For this review, take the finished solid that the model builds, in its own axes (mm). Face numbers are marked on the shaded views. A direction names the side the tool comes from. Coordinates: 2 decimals unless noted, no trailing zeros. Write each loop counter-clockwise with the first axis right and the second up, starting at its lowest first coordinate (ties: lowest second). Pieces come first, ordered by that corner, then holes. Notation, with made-up numbers: (-5, 55.25) - (48, 55.25) arc R32 cw to (48, 89.25) - close; hole circle Ø4 at (66.5, 37). An arc over 180 degrees is marked (long way). Use one line per item in the form item = value. Start each with the question number.
1) For L1, parallel to Z at x = 3, y = -15; L2, parallel to Y at x = 13.5, z = 10; L3, parallel to X at y = -20.5, z = 15, list the stretches that pass through material, from the lowest coordinate up. Write a range as from..to.
2) Insertion check: P1, Ø8, axis at x = -6, y = -0.5, coming from the -Z side; P2, Ø2, axis at x = 3, y = 8.5, coming from the +Z side; P3, Ø5, axis at y = -1.5, z = 18, coming from the +X side; P4, Ø5, axis at y = 12, z = 29, coming from the -X side. Each pin has a flat end and moves straight along its axis. Give the tip position at first contact, or say it passes through.
3) Mouldability with a two-part tool opening along Y and no side actions: class the marked faces 1, 2, 3 and 4 as pulls with the +Y half, pulls with the -Y half, needs draft (parallel to the pull), parting line crosses it, or undercut.
4) Tool access review of the marked faces 5, 6, 7 and 8: name each direction out of +Z, -Z, +X, -X, +Y, -Y from which nothing blocks a thin tool from reaching the whole face with its end or side.
5) We need section C-C (x = 0). Give the boundary of the cut face in (y, z), plus the area to 3 significant figures.
6) We need section D-D (z = 14.5). Give the boundary of the cut face in (x, y).
7) We need section B-B (z = 22.5). Give the boundary of the cut face in (x, y), plus the area to 3 significant figures.
8) We need section A-A (z = 35). Give the boundary of the cut face in (x, y).
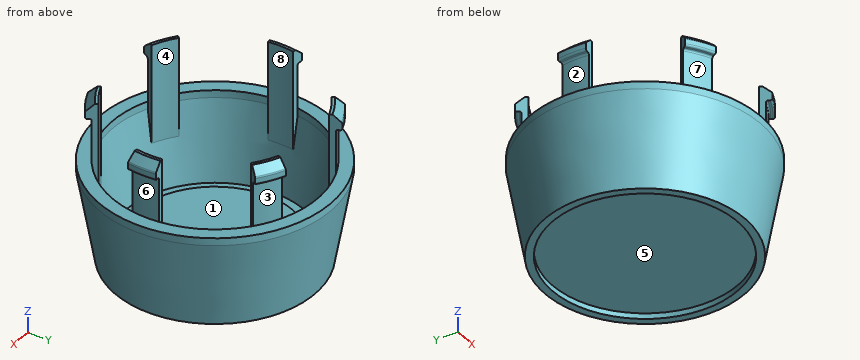
```python
from build123d import *

# Parameters (mm, degrees)
F3_ANGLE_BACK   = 7.5
F3_ANGLE        = 15
F3_COPIES_COUNT = 6
F4_R            = 0.5


# Not quite as in the source:
# - a pattern or mirror of a feature is missing from the dataset's text; its kind, count and spacing are read off the source's solid


with BuildPart() as f1:
    # F0 (on Front) → F1 (revolve)
    with BuildSketch(Plane.XZ):
        Polygon((-24.768152463, 1.5), (0, 1.5), (0, 4.5), (-20.8852968955, 4.5), (-20.8852968955, 3.5), (-23.8852968955, 3.5), (-27.5, 24), (-27.5, 26), (-31, 26), (-31, 24), (-26.768152463, 0), (-24.768152463, 0), align=None)
    revolve(axis=Axis((0, 0, 25), (0, 0, 1)))

    # F2 (on Front) → F3 (revolve)
    with BuildSketch(Plane.XZ, mode=Mode.PRIVATE) as f3_sk:
        Polygon((-27.5, 38), (-27.5, 24), (-26, 15.4930772706), (-26, 42), (-26.75, 42), (-29, 40), (-29, 38), align=None)
    f3 = revolve(f3_sk.sketch.rotate(Axis((0, 0, 25), (0, 0, 1)), -F3_ANGLE_BACK), axis=Axis((0, 0, 25), (0, 0, 1)), revolution_arc=F3_ANGLE)

    # F3_copies: F3 ×6 about axis
    f3_copies_axis = Axis((0, 0, 0), (0, 0, 1))
    for i in range(1, F3_COPIES_COUNT):
        add(f3.rotate(f3_copies_axis, i * 360 / F3_COPIES_COUNT))

    # F4
    f4_edges = [f1.edges().sort_by_distance(p)[0] for p in [
        (-29, 0, 38),
        (-29, 0, 40),
        (-27.5, 0, 38),
        (-13.75, -23.815699, 38),
        (13.75, -23.815699, 38),
        (27.5, 0, 38),
        (13.75, 23.815699, 38),
        (-13.75, 23.815699, 38),
        (-14.5, -25.114737, 38),
        (14.5, -25.114737, 38),
        (29, 0, 38),
        (14.5, 25.114737, 38),
        (-14.5, 25.114737, 38),
        (-14.5, -25.114737, 40),
        (14.5, -25.114737, 40),
        (29, 0, 40),
        (14.5, 25.114737, 40),
        (-14.5, 25.114737, 40),
    ]]
    fillet(f4_edges, radius=F4_R)


solid = f1.part
```
Determined:
q1.L1 = 1.5..4.5
q1.L2 = -25.14..-21.08, 21.08..25.14
q1.L3 = -21.09..-15.85, 15.85..21.09
q2.P1 = 1.5
q2.P2 = 4.5
q2.P3 = 30.36
q2.P4 = through
q3.face_1 = undercut
q3.face_2 = parting line crosses it
q3.face_3 = pulls with the +Y half
q3.face_4 = undercut
q4.face_5 = -Z
q4.face_6 = +X
q4.face_7 = -X, -Y
q4.face_8 = +Z
q5.outline = (-31, 24) - (-26.77, 0) - (-24.77, 0) - (-24.77, 1.5) - (24.77, 1.5) - (24.77, 0) - (26.77, 0) - (31, 24) - (31, 26) - (27.5, 26) - (27.5, 24) - (23.89, 3.5) - (20.89, 3.5) - (20.89, 4.5) - (-20.89, 4.5) - (-20.89, 3.5) - (-23.89, 3.5) - (-27.5, 24) - (-27.5, 26) - (-31, 26) - close
q5.area = 315 mm²
q6.outline = circle Ø58.65 at (0, 0); hole circle Ø51.65 at (0, 0)
q7.outline = circle Ø61.47 at (0, 0); hole (-27, -3.55) arc R27.24 ccw to (-16.58, -21.61) - (-15.83, -20.63) arc R26 ccw to (-9.95, -24.02) - (-10.42, -25.16) arc R27.24 ccw to (10.42, -25.16) - (9.95, -24.02) arc R26 ccw to (15.83, -20.63) - (16.58, -21.61) arc R27.24 ccw to (27, -3.55) - (25.78, -3.39) arc R26 ccw to (25.78, 3.39) - (27, 3.55) arc R27.24 ccw to (16.58, 21.61) - (15.83, 20.63) arc R26 ccw to (9.95, 24.02) - (10.42, 25.16) arc R27.24 ccw to (-10.42, 25.16) - (-9.95, 24.02) arc R26 ccw to (-15.83, 20.63) - (-16.58, 21.61) arc R27.24 ccw to (-27, 3.55) - (-25.78, 3.39) arc R26 ccw to (-25.78, -3.39) - close
q7.area = 689 mm²
q8.outline = (-27.26, -3.59) - (-25.78, -3.39) arc R26 cw to (-25.78, 3.39) - (-27.26, 3.59) arc R27.5 ccw to start; (-16.74, -21.82) arc R27.5 ccw to (-10.52, -25.41) - (-9.95, -24.02) arc R26 cw to (-15.83, -20.63) - close; (-16.74, 21.82) - (-15.83, 20.63) arc R26 cw to (-9.95, 24.02) - (-10.52, 25.41) arc R27.5 ccw to start; (9.95, -24.02) - (10.52, -25.41) arc R27.5 ccw to (16.74, -21.82) - (15.83, -20.63) arc R26 cw to start; (9.95, 24.02) arc R26 cw to (15.83, 20.63) - (16.74, 21.82) arc R27.5 ccw to (10.52, 25.41) - close; (25.78, -3.39) - (27.26, -3.59) arc R27.5 ccw to (27.26, 3.59) - (25.78, 3.39) arc R26 cw to start
